Check sheet for the modelled part. Datum: model origin and axes. Units: mm. A direction names the side the tool comes from. Coordinates: 2 decimals unless noted, no trailing zeros. Order: outer loops, then holes, each group sorted by start corner. A loop starts at its lowest first (then second) coordinate and runs counter-clockwise, first axis right, second up.
from build123d import *

# Parameters (mm, degrees)
F0_W     = 78.5
F0_H     = 94
F0_R     = 1.55
F0_R_2   = 4.25
F1_DEPTH = 3


with BuildPart() as f1:
    # F0 (on Front) → F1 (new body)
    with BuildSketch(Plane.XZ):
        with Locations((0, -0.289606)):
            Rectangle(F0_W, F0_H)
        with Locations((-35.3, -42.289606)):
            Circle(F0_R, mode=Mode.SUBTRACT)
        with Locations((35.3, -42.289606)):
            Circle(F0_R, mode=Mode.SUBTRACT)
        with BuildLine():
            Line((-24.249606, -34.007632), (-1.907053, -7.253492))
            ThreePointArc((-1.907053, -7.253492), (0, -7.5), (1.907053, -7.253492))
            Line((1.907053, -7.253492), (24.249606, -34.007632))
            ThreePointArc((24.249606, -34.007632), (24.526125, -36.13697), (22.714503, -37.289606))
            Line((22.714503, -37.289606), (-22.714503, -37.289606))
            ThreePointArc((-22.714503, -37.289606), (-24.526125, -36.13697), (-24.249606, -34.007632))
        make_face(mode=Mode.SUBTRACT)
        with BuildLine():
            Line((-29.25, -25.119712), (-29.25, 24.540499))
            ThreePointArc((-29.25, 24.540499), (-27.931833, 26.420686), (-25.714897, 25.822474))
            Line((-25.714897, 25.822474), (-6.79733, 3.169591))
            ThreePointArc((-6.79733, 3.169591), (-7.497264, -0.202557), (-6.61627, -3.531993))
            Line((-6.61627, -3.531993), (-25.714897, -26.401686))
            ThreePointArc((-25.714897, -26.401686), (-27.931833, -26.999899), (-29.25, -25.119712))
        make_face(mode=Mode.SUBTRACT)
        with Locations((-35.3, 41.710394)):
            Circle(F0_R, mode=Mode.SUBTRACT)
        Circle(F0_R_2, mode=Mode.SUBTRACT)
        with BuildLine():
            ThreePointArc((6.61627, -3.531993), (7.497264, -0.202557), (6.79733, 3.169591))
            Line((6.79733, 3.169591), (25.714897, 25.822474))
            ThreePointArc((25.714897, 25.822474), (27.931833, 26.420686), (29.25, 24.540499))
            Line((29.25, 24.540499), (29.25, -25.119712))
            ThreePointArc((29.25, -25.119712), (27.931833, -26.999899), (25.714897, -26.401686))
            Line((25.714897, -26.401686), (6.61627, -3.531993))
        make_face(mode=Mode.SUBTRACT)
        with BuildLine():
            ThreePointArc((-24.249606, 33.428419), (-24.526125, 35.557758), (-22.714503, 36.710394))
            Line((-22.714503, 36.710394), (22.714503, 36.710394))
            ThreePointArc((22.714503, 36.710394), (24.526125, 35.557758), (24.249606, 33.428419))
            Line((24.249606, 33.428419), (2.295928, 7.139938))
            ThreePointArc((2.295928, 7.139938), (0, 7.5), (-2.295928, 7.139938))
            Line((-2.295928, 7.139938), (-24.249606, 33.428419))
        make_face(mode=Mode.SUBTRACT)
        with Locations((35.3, 41.710394)):
            Circle(F0_R, mode=Mode.SUBTRACT)
    extrude(amount=F1_DEPTH)


solid = f1.part
(1) Release check for a two-part mould opening along Z. For faces 3 (the cylindrical face through (24.54, -1.48, -36.11)), 4 (the flat face through (-1, -1, -47.29)), 5 (the flat face through (-39.25, -1, -1)) record: +Z half, -Z half, draft (parallel to the pull), parting line (faces both ways), or undercut.
Filled in:
face 3: undercut
face 4: -Z half
face 5: draft
(2) Thickness scan on probe 1 along Z at (x, y) = (-35.3, -2.3); probe 2 along X at (y, z) = (-1.5, -41); probe 3 along Z at (x, y) = (-11.5, -1.7). Record the ranges inside material, lowest first.
Filled in:
probe 1: z = -47.29 to -43.84, -40.74 to 40.16, 43.26 to 46.71
probe 2: x = -39.25 to -36.16, -34.44 to 34.44, 36.16 to 39.25
probe 3: z = -47.29 to -37.29, -18.74 to -9.38, 8.8 to 18.16, 36.71 to 46.71
(3) Cross-section at D-D (y = -1.95). Count the separate pieces of the cut face and the enclosed holes in it, and give its area (3 significant figures).
Filled in:
separate pieces: 1
enclosed holes: 9
area: 4,090 mm2
(4) Cross-section at C-C (x = -35.3). Enter the section's corners in (y, z).
Filled in:
outline: (-3, -47.29) - (0, -47.29) - (0, -43.84) - (-3, -43.84) - close; (-3, -40.74) - (0, -40.74) - (0, 40.16) - (-3, 40.16) - close; (-3, 43.26) - (0, 43.26) - (0, 46.71) - (-3, 46.71) - close
(5) Tool access check on faces 1 (the flat face through (0, -1, 36.71)), 2 (the flat face through (8, -3, 11)). Record the directions out of +Z, -Z, +X, -X, +Y, -Y that give a thin tool (end or side, any length) a straight path to the whole face; none if there is none.
Filled in:
face 1: +Y, -Y
face 2: +Z, -Z, +X, -X, -Y
(6) Cross-section at B-B (z = 0). Enter the section's corners in (x, y), and give its area (3 significant figures).
Filled in:
outline: (-39.25, -3) - (-29.25, -3) - (-29.25, 0) - (-39.25, 0) - close; (-7.5, -3) - (-4.25, -3) - (-4.25, 0) - (-7.5, 0) - close; (4.25, -3) - (7.5, -3) - (7.5, 0) - (4.25, 0) - close; (29.25, -3) - (39.25, -3) - (39.25, 0) - (29.25, 0) - close
area: 79.5 mm2
(7) Cross-section at A-A (x = 0). Enter the section's corners in (y, z).
Filled in:
outline: (-3, -47.29) - (0, -47.29) - (0, -37.29) - (-3, -37.29) - close; (-3, -7.5) - (0, -7.5) - (0, -4.25) - (-3, -4.25) - close; (-3, 4.25) - (0, 4.25) - (0, 7.5) - (-3, 7.5) - close; (-3, 36.71) - (0, 36.71) - (0, 46.71) - (-3, 46.71) - close
(8) Go/stop test with a flat-tipped pin: P1, Ø2, axis at x = -4, z = 12, coming from the -Y side. Record where the tip stops, or that it passes through.
Filled in:
P1: passes through
